from build123d import *

# Parameters (mm, degrees)
SKETCH1_R           = 2.25
SKETCH1_R_2         = 1
BOSS_EXTRUDE1_DEPTH = 6
SKETCH2_R           = 1.5
SKETCH2_R_2         = 1
BOSS_EXTRUDE2_DEPTH = 1.5
SKETCH3_R           = 2.25
SKETCH3_R_2         = 1
BOSS_EXTRUDE3_DEPTH = 1.5


with BuildPart() as part:
    # Sketch1 → Boss-Extrude1 (new body)
    with BuildSketch(Plane(origin=(0, 0, 0), x_dir=(1, 0, 0), z_dir=(0, 1, 0))):
        Circle(SKETCH1_R)
        Circle(SKETCH1_R_2, mode=Mode.SUBTRACT)
    extrude(amount=BOSS_EXTRUDE1_DEPTH)

    # Sketch2 → Boss-Extrude2 (add)
    with BuildSketch(Plane(origin=(0, 6, 0), x_dir=(1, 0, 0), z_dir=(0, 1, 0))):
        Circle(SKETCH2_R)
        Circle(SKETCH2_R_2, mode=Mode.SUBTRACT)
    extrude(amount=BOSS_EXTRUDE2_DEPTH)

    # Sketch3 → Boss-Extrude3 (add)
    with BuildSketch(Plane(origin=(0, 7.5, 0), x_dir=(1, 0, 0), z_dir=(0, 1, 0))):
        Circle(SKETCH3_R)
        Circle(SKETCH3_R_2, mode=Mode.SUBTRACT)
    extrude(amount=BOSS_EXTRUDE3_DEPTH)


solid = part.part
The listing builds one solid part. Answer for the finished solid, in the listing's coordinates (mm). A direction names the side the tool comes from. Coordinates: 2 decimals unless noted, no trailing zeros. Write each loop counter-clockwise with the first axis right and the second up, starting at its lowest first coordinate (ties: lowest second). Pieces come first, ordered by that corner, then holes. Notation, with made-up numbers: M 86.5,-20.5 L 101.5,-20.5 A22 ccw 101.5,1.5 Z; hole C 48,-30.75 d9. An arc over 180 degrees is marked long. Write each question's results on one line, items separated by ' | '.
Item 1: The part is cut by section A-A on x = 0. Determine the outline of the cut face in (y, z), and give its area (4 significant figures).
Answer below:
outline: M 0,-2.25 L 6,-2.25 L 6,-1.5 L 7.5,-1.5 L 7.5,-2.25 L 9,-2.25 L 9,-1 L 0,-1 Z; M 0,1 L 9,1 L 9,2.25 L 7.5,2.25 L 7.5,1.5 L 6,1.5 L 6,2.25 L 0,2.25 Z | area: 20.25 mm2
Item 2: For a pull along Y with two mould halves and no side action, classify faces 1 (the face through (-1.5, 6.74, -0.07)), 2 (the face through (-0.29, 2.96, -2.23)), 3 (the face through (-1, 9, 1)), 4 (the face through (-1, 0, 1)) as released by +Y, released by -Y, zero draft, split by the parting line, or undercut.
Answer below:
face 1: undercut | face 2: zero draft | face 3: released by +Y | face 4: released by -Y
Item 3: Which of the six approach directions +Z, -Z, +X, -X, +Y, -Y give full straight-line access (tool end or side, diameter ignored) to faces 5 (the face through (0, 4, 1)), 6 (the face through (-2, 6, 0))?
Answer below:
face 5: +Y, -Y | face 6: none
Item 4: Consider probe 1 along Y at (x, z) = (0.8, -1.9); probe 2 along Z at (x, y) = (0, 2). Determine where each line is inside the solid, lowest interval first. Write a range as [from, to].
Answer below:
probe 1: [0, 6], [7.5, 9] | probe 2: [-2.25, -1], [1, 2.25]
Item 5: The part is cut by section C-C on y = 5. Determine the outline of the cut face in (x, z), and give its area (3 significant figures).
Answer below:
outline: C 0,0 d4.5; hole C 0,0 d2 | area: 12.8 mm2
Item 6: Given P1, Ø1.5, axis at y = 3.5, z = 1, coming from the +X side, flat-ended and moving along its own axis, determine where the tip first touches the part or whether it passes through.
Answer below:
P1: x = 2.24
Item 7: The part is cut by section B-B on z = 0. Determine the outline of the cut face in (x, y), and give its area (4 significant figures).
Answer below:
outline: M -2.25,0 L -1,0 L -1,9 L -2.25,9 L -2.25,7.5 L -1.5,7.5 L -1.5,6 L -2.25,6 Z; M 1,0 L 2.25,0 L 2.25,6 L 1.5,6 L 1.5,7.5 L 2.25,7.5 L 2.25,9 L 1,9 Z | area: 20.25 mm2
Item 8: The part is cut by section D-D on z = -1.4. Determine the outline of the cut face in (x, y).
Answer below:
outline: M -1.76,0 L 1.76,0 L 1.76,6 L 0.54,6 L 0.54,7.5 L 1.76,7.5 L 1.76,9 L -1.76,9 L -1.76,7.5 L -0.54,7.5 L -0.54,6 L -1.76,6 Z
